```python
from build123d import *

# Parameters (mm, degrees)
CUT_EXTRUDE1_DEPTH = 10


with BuildPart() as part:
    # Sketch1 → Revolve1 (revolve)
    with BuildSketch(Plane.XY):
        with BuildLine():
            Line((0, 0), (0, -25))
            Line((0, -25), (2.5, -25))
            Line((2.5, -25), (2.5, 0))
            Line((2.5, 0), (4.65, 0))
            ThreePointArc((4.65, 0), (2.713968497, 2.045965539), (0, 2.8))
            Line((0, 2.8), (0, 0))
        make_face()
    revolve(axis=Axis((0, 0, 0), (0, -1, 0)))

    # Sketch2 → Cut-Extrude1 (cut)
    with BuildSketch(Plane(origin=(0, 0, 0), x_dir=(1, 0, 0), z_dir=(0, 1, 0))):
        Polygon((0, 1.732050808), (-1.5, 0.866025404), (-1.5, -0.866025404), (0, -1.732050808), (1.5, -0.866025404), (1.5, 0.866025404), align=None)
    extrude(amount=CUT_EXTRUDE1_DEPTH, mode=Mode.SUBTRACT)


solid = part.part
```
Geometry: final body of the model. Coordinates: model frame, mm. A direction names the side the tool comes from. Coordinates: 2 decimals unless noted, no trailing zeros. Order: outer loops, then holes, each group sorted by start corner. A loop starts at its lowest first (then second) coordinate and runs counter-clockwise, first axis right, second up. Notation, with made-up numbers: M 41.25,75.5 L 94.25,75.5 A19 cw 94.25,93.5 Z; hole C -15.75,-32 d5. An arc over 180 degrees is marked long. Answer in a Markdown table with one row per item. Add a question column.
Q1. Mould query, pull axis X, two halves, no side actions, for faces 3 (the flat face through (0.761, 1.273, -1.293)), 4 (the cylindrical face through (-0.54, -12.32, -2.44)), 5 (the flat face through (0, -25, 0)). Classes: released by +X, released by -X, zero draft, split by the parting line, or undercut.
Q2. Reachability of faces 1 (the flat face through (-0.761, 1.273, 1.293)), 2 (the flat face through (-2, 0, -2)) from +Z, -Z, +X, -X, +Y, -Y: full face, straight path, thin tool, end or side. Return the list, or none.
Q3. Section query C-C on y = -20.5. Return the cut outline in (x, z).
Q4. Section query D-D on z = 3.25. Return the cut outline in (x, y), and give its area (3 significant figures).
Q5. Section query B-B on x = 0.5. Return the cut outline in (y, z).
Q6. Line query: L1, parallel to Y at x = 2.75, z = 0; L2, parallel to Z at x = 0.5, y = -8.5; L3, parallel to Z at x = -1.75, y = -0.25. Output: solid intervals per line, ascending.
Q7. Contact query for flat-ended pins moving along their axis: P1, Ø5, axis at x = 3.5, y = -17, coming from the +Z side; P2, Ø1.9, axis at y = 2, z = 0, coming from the -X side; P3, Ø3, axis at x = 2, y = -17, coming from the -Z side. Output: stop coordinate, or through.
Q8. Section query A-A on z = 0. Return the cut outline in (x, y), and give its area (3 significant figures).
Completed:
| question | item | result |
|---|---|---|
| 1 | face 3 | undercut |
| 1 | face 4 | split by the parting line |
| 1 | face 5 | zero draft |
| 2 | face 1 | +Y |
| 2 | face 2 | -Y |
| 3 | outline | C 0,0 d5 |
| 4 | outline | M -3.33,0 L 3.33,0 A4.14 ccw Z |
| 4 | area | 7.80 mm2 |
| 5 | outline | M -25,-2.45 L 0,-2.45 L 0,-4.62 A5.24 ccw 2.57,-1.44 L 0,-1.44 L 0,1.44 L 2.57,1.44 A5.24 ccw 0,4.62 L 0,2.45 L -25,2.45 Z |
| 6 | L1 | y = 0 to 2.02 |
| 6 | L2 | z = -2.45 to 2.45 |
| 6 | L3 | z = -1.79 to 1.79 |
| 7 | P1 | stops at z = 2.29 |
| 7 | P2 | stops at x = -3.92 |
| 7 | P3 | stops at z = -2.45 |
| 8 | outline | M -4.65,0 L -2.5,0 L -2.5,-25 L 2.5,-25 L 2.5,0 L 4.65,0 A5.26 ccw 1.5,2.58 L 1.5,0 L -1.5,0 L -1.5,2.58 A5.26 ccw Z |
| 8 | area | 135 mm2 |
